Build history of the part. All positions in model axes, mm. Face numbers are marked on the shaded views. A direction names the side the tool comes from. Give positions to 0.01 mm unless a question says otherwise; leave off trailing zeros. Order: outer loops, then holes, each group sorted by start corner. A loop starts at its lowest first (then second) coordinate and runs counter-clockwise, first axis right, second up. Notation, with made-up numbers: (2.5, -18.75) -> (44.5, -18.75) arc R24 cw to (44.5, -1.75) -> close; hole circle Ø2 at (42.5, -32.5). An arc over 180 degrees is marked (long way). Use a Markdown table: item, result. Add a question column.
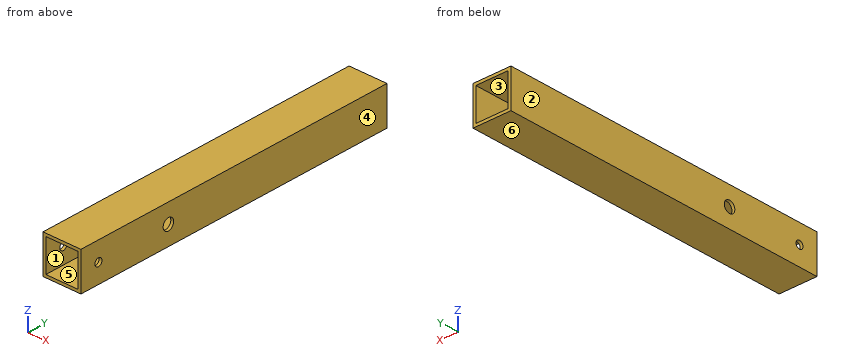
```python
from build123d import *

# Parameters (mm, degrees)
F0_W     = 20
F0_H     = 20
F0_W_2   = 17
F0_H_2   = 17
F1_DEPTH = 175
F3_D     = 4
F5_D     = 6


with BuildPart() as f1:
    # F0 (on Front) → F1 (new body)
    with BuildSketch(Plane.XZ):
        Rectangle(F0_W, F0_H)
        Rectangle(F0_W_2, F0_H_2, mode=Mode.SUBTRACT)
    extrude(amount=F1_DEPTH)

    # F3 (through all)
    with Locations(Plane.YZ.offset(10)):
        with Locations((-165, 0)):
            Hole(F3_D / 2)

    # F5 (through all)
    with Locations(Plane.YZ.offset(10)):
        with Locations((-125, 0)):
            Hole(F5_D / 2)


solid = f1.part
```
(1) Tool access for the marked faces 5 and 6: list every direction of +Z, -Z, +X, -X, +Y, -Y with a clear straight run to the whole face (end or side of a thin tool).
(2) Band-saw the part on B-B on y = -31. Give the cut face in (x, z), plus the area to 3 significant figures.
(3) Pin check, flat tip, straight feed: pin 1 Ø3 at (y, z) = (-165, 0) entering from -X. Stop position of the tip, or through.
(4) Band-saw the part on A-A on z = 0. Give the cut face in (x, y).
(5) Mould opens along X. For the marked faces 1, 2, 3 and 4 say: released by +X, released by -X, zero draft, split by the parting line, or undercut.
(6) Band-saw the part on D-D on y = -165. Give the cut face in (x, z), plus the area to 3 significant figures.
(7) Band-saw the part on C-C on x = -1.5. Give the cut face in (y, z).
(8) Wall check: probe 1 along X at (y, z) = (-147.5, -0.5); probe 2 along Z at (x, y) = (-9.05, -165); probe 3 along Z at (x, y) = (9.3, -125). Give the ranges that are in metal, low to high.
Response:
| question | item | result |
|---|---|---|
| 1 | face 5 | +Y, -Y |
| 1 | face 6 | -Z, +X, -X, +Y, -Y |
| 2 | outline | (-10, -10) -> (10, -10) -> (10, 10) -> (-10, 10) -> close; hole (-8.5, -8.5) -> (8.5, -8.5) -> (8.5, 8.5) -> (-8.5, 8.5) -> close |
| 2 | area | 111 mm² |
| 3 | pin 1 | passes through |
| 4 | outline | (-10, -175) -> (-8.5, -175) -> (-8.5, -167) -> (-10, -167) -> close; (-10, -163) -> (-8.5, -163) -> (-8.5, -128) -> (-10, -128) -> close; (-10, -122) -> (-8.5, -122) -> (-8.5, 0) -> (-10, 0) -> close; (8.5, -175) -> (10, -175) -> (10, -167) -> (8.5, -167) -> close; (8.5, -163) -> (10, -163) -> (10, -128) -> (8.5, -128) -> close; (8.5, -122) -> (10, -122) -> (10, 0) -> (8.5, 0) -> close |
| 5 | face 1 | undercut |
| 5 | face 2 | released by -X |
| 5 | face 3 | undercut |
| 5 | face 4 | released by +X |
| 6 | outline | (-10, -10) -> (10, -10) -> (10, -2) -> (8.5, -2) -> (8.5, -8.5) -> (-8.5, -8.5) -> (-8.5, -2) -> (-10, -2) -> close; (-10, 2) -> (-8.5, 2) -> (-8.5, 8.5) -> (8.5, 8.5) -> (8.5, 2) -> (10, 2) -> (10, 10) -> (-10, 10) -> close |
| 6 | area | 99.0 mm² |
| 7 | outline | (-175, -10) -> (0, -10) -> (0, -8.5) -> (-175, -8.5) -> close; (-175, 8.5) -> (0, 8.5) -> (0, 10) -> (-175, 10) -> close |
| 8 | probe 1 | x = -10 to -8.5, 8.5 to 10 |
| 8 | probe 2 | z = -10 to -2, 2 to 10 |
| 8 | probe 3 | z = -10 to -3, 3 to 10 |
